Autodesk Inventor part; units mm, degrees
ref_plane "YZ Plane" through (0, 0, 0) normal (1, 0, 0) x (0, 1, 0)
ref_plane "XZ Plane" through (0, 0, 0) normal (0, 1, 0) x (-1, 0, 0)
ref_plane "XY Plane" through (0, 0, 0) normal (0, 0, 1) x (1, 0, 0)
sketch "Sketch1" plane through (0, 0, 0) normal (0, 0, 1) x (1, 0, 0)
  line L0 (-4.7625, 12.7) -> (4.7625, 12.7)
  line L1 (4.7625, 12.7) -> (4.7625, -12.7)
  line L2 (4.7625, -12.7) -> (-4.7625, -12.7)
  line L3 (-4.7625, -12.7) -> (-4.7625, 12.7)
  line L4 (-4.7625, 12.7) -> (4.7625, -12.7) construction
  line L5 (4.7625, 12.7) -> (-4.7625, -12.7) construction
  circle A0 centre (1.5875, 0) radius 2.5527
  line L6 (1.5875, 2.5527) -> (4.7625, 2.5527)
  line L7 (1.5875, -2.5527) -> (4.7625, -2.5527)
  point P0 (0, 0)
  dimension "d0" = 9.525
  dimension "d1" = 25.4
  dimension "d2" = 3.175
  dimension "d3" = 12.7
  dimension "d4" = 5.1054
extrude "Extrusion1" add sketch "Sketch1" along normal blind 12.7 contours L0 L1 L6 A0 L7 L2 L3
fillet "Fillet1" radius 3.175 4 edges at (-4.7625, 12.7, 6.35) (4.7625, 12.7, 6.35) (4.7625, -12.7, 6.35) (-4.7625, -12.7, 6.35)
properties part number "CANdle spacer" material "ABS Plastic"
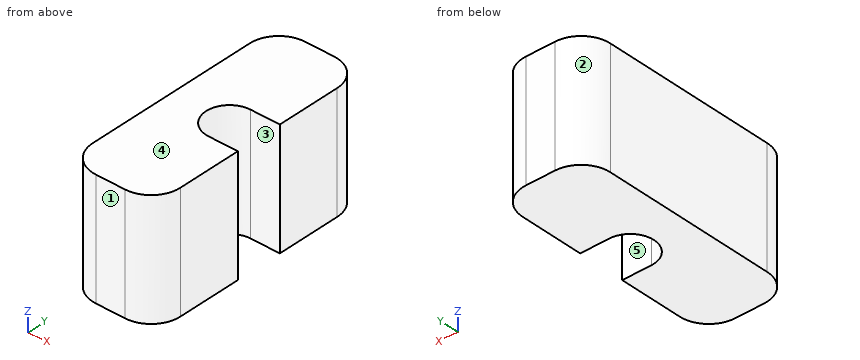
Check sheet for the modelled part. Datum: model origin and axes. Units: mm. Face numbers are marked on the shaded views. A direction names the side the tool comes from. Round coordinates to 2 decimals unless told otherwise and drop trailing zeros. Order: outer loops, then holes, each group sorted by start corner. A loop starts at its lowest first (then second) coordinate and runs counter-clockwise, first axis right, second up. Notation, with made-up numbers: M 56,74.25 L 93,74.25 A25 ccw 93,95.25 Z; hole C 49,88.5 d4. An arc over 180 degrees is marked long. One line per item, written item: value. Start each with the question number.
1. Section check C-C on y = 0. Enter the section's corners in (x, z).
2. Gauge pin test, flat ends, axial feed: P1, Ø1, axis at x = 3.5, z = 6, coming from the +Y side; P2, Ø1, axis at x = 3, z = 6, coming from the +Y side; P3, Ø1, axis at x = -3.5, z = 2.5, coming from the -Y side; P4, Ø2.5, axis at x = 2.5, z = 4.5, coming from the -Y side. Record the tip position at first contact, or that the pin passes through.
3. Section check A-A on x = 3.5. Enter the section's corners in (y, z).
4. Access from +Z, -Z, +X, -X, +Y, -Y to the whole of each face (thin tool, end or side, straight path). Record for the marked faces 4 and 5.
5. Scan lines: line 1 along Y through (x, z) = (1.5, 9); line 2 along Y through (x, z) = (0.5, 7.5); line 3 along X through (y, z) = (0, 1.5). Record each from-to range of solid material in increasing order.
6. Release check for a two-part mould opening along Y. For the marked faces 1, 2 and 3 record: released by +Y, released by -Y, zero draft, split by the parting line, or undercut.
Results found:
1. outline: M -4.76,0 L -0.97,0 L -0.97,12.7 L -4.76,12.7 Z
2. P1: y = 12.37
2. P2: y = 12.57
2. P3: y = -12.37
2. P4: y = -12.7
3. outline: M -12.06,0 L -2.55,0 L -2.55,12.7 L -12.06,12.7 Z; M 2.55,0 L 12.06,0 L 12.06,12.7 L 2.55,12.7 Z
4. face 4: +Z, +X, -X, +Y, -Y
4. face 5: +Z, -Z, +X
5. line 1: -12.7 to -2.55, 2.55 to 12.7
5. line 2: -12.7 to -2.31, 2.31 to 12.7
5. line 3: -4.76 to -0.97
6. face 1: released by -Y
6. face 2: released by +Y
6. face 3: undercut
